Check sheet for the modelled part. Datum: model origin and axes. Units: mm. A direction names the side the tool comes from. Give positions to 0.01 mm unless a question says otherwise; leave off trailing zeros. Loops run counter-clockwise (first coordinate to the right, second up) from the corner with the lowest first, then second, coordinate; pieces in that order, holes last. Notation, with made-up numbers: M -36,47.5 L -10,47.5 A19 ccw -10,82.5 Z; hole C 4.25,15.5 d6. An arc over 180 degrees is marked long. Use one line per item in the form item = value.
Autodesk Inventor part; units mm, degrees
ref_plane "Arbeitsebene_Bohrung" through (-29.0381, -10, 45.9619) normal (-0.7071068, 0, 0.7071068) x (0.7071068, 0, 0.7071068)
ref_plane "YZ Plane" through (0, 0, 0) normal (1, 0, 0) x (0, 1, 0)
ref_plane "XZ Plane" through (0, 0, 0) normal (0, 1, 0) x (-1, 0, 0)
sketch "Skizze1" plane through (0, 0, 0) normal (0, 1, 0) x (-1, 0, 0)
  line L0 (75, 0) -> (-5, 80) construction
  line L1 (5, 80) -> (-75, 0) construction
  line L2 (75, 21.2132) -> (39.6447, 56.5685)
  line L3 (39.6447, 56.5685) -> (18.4315, 35.3553)
  line L4 (18.4315, 35.3553) -> (53.7868, 0)
  line L5 (-18.4315, 35.3553) -> (-39.6447, 56.5685)
  line L6 (-39.6447, 56.5685) -> (-75, 21.2132)
  line L7 (-18.4315, 35.3553) -> (-53.7868, 0)
  line L8 (75, 38.1838) -> (33.1838, 80)
  line L9 (-75, 38.1838) -> (-33.1838, 80)
  line L10 (8.8388, 27.9774) -> (36.8162, 0)
  line L11 (-8.8388, 27.9774) -> (-36.8162, 0)
  arc A0 (8.8388, 27.9774) -> (-8.8388, 27.9774) centre (0, 19.1386) ccw
  line L12 (-33.1838, 80) -> (33.1838, 80)
  line L13 (53.7868, 0) -> (36.8162, 0)
  line L14 (-36.8162, 0) -> (-53.7868, 0)
  line L15 (-75, 21.2132) -> (-75, 38.1838)
  line L16 (75, 21.2132) -> (75, 38.1838)
  line L17 (0, -16) -> (0, 96) construction
  line L18 (-105, 0) -> (105, 0) construction
  line L19 (39.6447, 56.5685) -> (48.1299, 65.0538)
  point P0 (0, 36.8162)
  point P1 (0, 0)
  dimension "d11" = 30
  dimension "d12" = 50
  dimension "d16" = 12
  dimension "d17" = 12
  dimension "d18" = 12.5
  dimension "d19" = 80
  dimension "d20" = 150
  dimension "d21" = 45
extrude "Grundkörper" add sketch "Skizze1" along normal mid plane 20
sketch "Skizze2" plane through (0, 10, 0) normal (0, 1, 0) x (1, 0, 0)
  line L0 (0, 16) -> (0, -96) construction
  line L1 (-33.1838, -80) -> (33.1838, -80) construction
  line L2 (105, 0) -> (-105, 0) construction
  line L3 (10, -80) -> (-10, -80)
  line L4 (-10, -80) -> (-10, 0)
  line L5 (-10, 0) -> (10, 0)
  line L6 (10, 0) -> (10, -80)
  point P0 (0, 0)
  dimension "d25" = 20
extrude "NUT" cut sketch "Skizze2" against normal blind 5
sketch "Skizze4" plane through (0, -10, 0) normal (0, -1, 0) x (1, 0, 0)
  line L0 (0, 96) -> (0, -16) construction
  line L1 (33.1838, 80) -> (-33.1838, 80) construction
  point P0 (0, 0)
  point P1 (0, 55)
  dimension "d29" = 25
hole "DIN7984_M8_Bohrung" at (0, -10, 55) direction (0, 1, 0) diameter 9 end through all counterbore diameter 15 counterbore depth 5.4
ref_plane "Arbeitsebene_Bohrung" through (-29.0381, -10, 45.9619) normal (-0.7071068, 0, 0.7071068) x (0.7071068, 0, 0.7071068)
sketch "Skizze5" plane through (-33.1838, -10, 80) normal (-0.7071068, 0, 0.7071068) x (0.7071068, 0, 0.7071068)
  line L0 (-21.1371, 20) -> (-21.1371, 0) construction
  line L1 (-59.1371, 20) -> (-59.1371, 0) construction
  line L2 (-125.864, 10) -> (110.2244, 10) construction
  line L3 (-71.1371, 0) -> (-71.1371, 20)
  point P0 (-33.1041, 10)
  point P1 (-33.1371, 10)
  point P2 (-53.1371, 10)
  dimension "d37" = 20
  dimension "d39" = 18
hole "DIN7984_M6_Bohrung" at (-56.6152, 0, 56.5685) at (-70.7574, 0, 42.4264) direction (0.7071068, 0, -0.7071068) diameter 6.6 end up to surface counterbore diameter 11 counterbore depth 4.4
mirror "DIN7984_M6_Bohrung_Spiegelung:1" about plane through (-29.0381, -10, 45.9619) normal (-0.7071068, 0, 0.7071068) of "DIN7984_M6_Bohrung"
mirror "DIN7984_M6_Bohrung_Spiegelung:2" about plane through (0, 0, 0) normal (1, 0, 0) of "DIN7984_M6_Bohrung", "DIN7984_M6_Bohrung_Spiegelung:1"
equation "\"d17\" = d16"
properties part number "200-20-ROCKER-CONNECTOR-03" material "Aluminium 6061"
1) Section check B-B (y = -7). Record the cut outline in (x, z).
Evaluation:
outline = M -75,21.21 L -39.64,56.57 L -18.43,35.36 L -53.79,0 L -36.82,0 L -8.84,27.98 A12.5 cw 8.84,27.98 L 36.82,0 L 53.79,0 L 18.43,35.36 L 39.64,56.57 L 75,21.21 L 75,38.18 L 33.18,80 L -33.18,80 L -75,38.18 Z; hole C 0,55 d15
2) Section check C-C (z = 69.5). Record the cut outline in (x, y), then the cut area to 3 significant figures.
Evaluation:
outline = M -43.68,-10 L 43.68,-10 L 43.68,10 L 10,10 L 10,5 L -10,5 L -10,10 L -43.68,10 Z
area = 1,650 mm^2
3) Scan lines: line 1 (X direction, y = -6.6, z = 55); line 2 (X direction, y = 6.5, z = 23); line 3 (X direction, y = 4, z = 37). Record each from-to range of solid material in increasing order.
Evaluation:
line_1 = -58.18 to -41.21, -38.08 to -7.5, 7.5 to 38.08, 41.21 to 58.18
line_2 = -75 to -73.21, -30.79 to -13.82, 13.82 to 30.79, 73.21 to 75
line_3 = -75 to -70.67, -69.96 to -59.21, -20.08 to 20.08, 59.21 to 69.96, 70.67 to 75
4) Release check for a two-part mould opening along Y. For faces 4 (the face through (21.6, -3.59, 21.44)), 5 (the face through (-75, 0, 30)), 6 (the face through (5, -4.6, 55)) record: pulls with the +Y half, pulls with the -Y half, needs draft (parallel to the pull), parting line crosses it, or undercut.
Evaluation:
face_4 = undercut
face_5 = needs draft
face_6 = pulls with the -Y half
5) Section check A-A (x = 0). Record the cut outline in (y, z).
Evaluation:
outline = M -10,31.64 L 5,31.64 L 5,50.5 L -4.6,50.5 L -4.6,47.5 L -10,47.5 Z; M -10,62.5 L -4.6,62.5 L -4.6,59.5 L 5,59.5 L 5,80 L -10,80 Z
6) Depth check by flat-ended pin: pin 1 Ø4 at (y, z) = (7, 65) entering from +X; pin 2 Ø4.5 at (x, z) = (-3.5, 55.5) entering from -Y; pin 3 Ø12 at (x, z) = (2, 35) entering from +Y; pin 4 Ø24 at (x, z) = (0, 55) entering from +Y. Enter the tip coordinate at first touch or a pass-through.
Evaluation:
pin_1 = 50.18
pin_2 = -4.6
pin_3 = 5
pin_4 = 10
7) Section check D-D (x = -52). State how many separate pieces and enclosed holes the cut face has, then the cut area to 3 significant figures.
Evaluation:
separate_pieces = 2
enclosed_holes = 1
area = 298 mm^2
8) Set-up check for faces 1 (the face through (-53.56, -3.59, 53.4)), 2 (the face through (-28, 10, 49)), 3 (the face through (-29.187, -0.14, 46.11)): record each of +Z, -Z, +X, -X, +Y, -Y from which the full face is reachable in a straight line by a thin tool's end or side.
Evaluation:
face_1 = none
face_2 = +Z, -Z, +X, -X, +Y
face_3 = +Y, -Y
